For this review, take the finished solid that the model builds, in its own axes (mm). Round coordinates to 2 decimals unless told otherwise and drop trailing zeros. Write each loop counter-clockwise with the first axis right and the second up, starting at its lowest first coordinate (ties: lowest second). Pieces come first, ordered by that corner, then holes. Notation, with made-up numbers: M 23.25,15.5 L 68.25,15.5 A12 cw 68.25,31.5 Z; hole C 59.5,47 d8. An arc over 180 degrees is marked long. One line per question, with ' | ' between items.
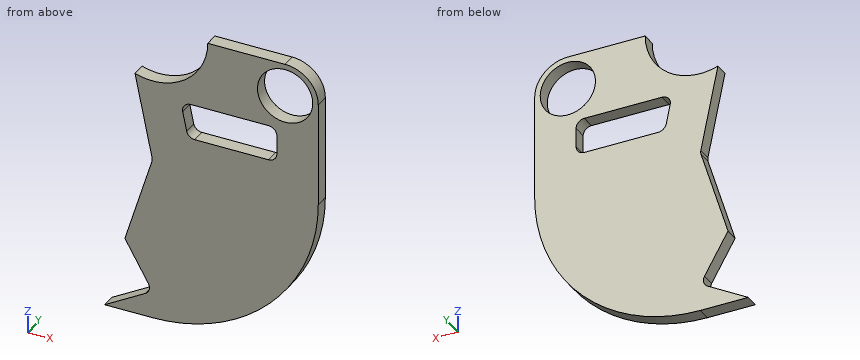
```python
from build123d import *

# Parameters (mm, degrees)
PROFILE_SKETCH_R      = 10
PROFILE_EXTRUDE_DEPTH = 5
TRAPEZOID_FILLET_R    = 3
CLAW_FILLET_R         = 3


with BuildPart() as part:
    # Profile Sketch → Profile Extrude (new body)
    with BuildSketch(Plane(origin=(0, 0, 0), x_dir=(1, 0, 0), z_dir=(0, 1, 0))):
        with BuildLine():
            Line((0, 60), (-17.320508076, 60))
            Line((-17.320508076, 60), (0, 50))
            Line((0, 50), (-10, 32.679491924))
            Line((-10, 32.679491924), (0, 0))
            Line((0, 0), (-6.333857356, -31.029437252))
            ThreePointArc((-6.333857356, -31.029437252), (11.690227818, -33.772289947), (20, -50))
            Line((20, -50), (48, -50))
            ThreePointArc((48, -50), (56.485281374, -46.485281374), (60, -38))
            Line((60, -38), (60, 0))
            ThreePointArc((60, 0), (42.426406871, 42.426406871), (0, 60))
        make_face()
        with Locations(Location((48, -38, 0), (0, 0, 270))):
            Circle(PROFILE_SKETCH_R, mode=Mode.SUBTRACT)
        Polygon((12.853812296, -12.029437252), (45, -12.029437252), (45, -25), (10.206207262, -25), align=None, mode=Mode.SUBTRACT)
    extrude(amount=PROFILE_EXTRUDE_DEPTH)

    # Trapezoid Fillet
    trapezoid_fillet_edges = [part.edges().sort_by_distance(p)[0] for p in [
        (10.206207262, 2.5, 25),
        (45, 2.5, 25),
        (45, 2.5, 12.029437252),
        (12.853812296, 2.5, 12.029437252),
    ]]
    fillet(trapezoid_fillet_edges, radius=TRAPEZOID_FILLET_R)

    # Claw Fillet
    claw_fillet_edges = [part.edges().sort_by_distance(p)[0] for p in [
        (0, 2.5, -50),
        (0, 2.5, 0),
    ]]
    fillet(claw_fillet_edges, radius=CLAW_FILLET_R)


solid = part.part
```
Item 1: Take a section at B-B (z = 19.5). Write out the cut boundary in (x, y), then the cut area to 3 significant figures.
Results:
outline: M -3.98,0 L 11.33,0 L 11.33,5 L -3.98,5 Z; M 45,0 L 60,0 L 60,5 L 45,5 Z | area: 152 mm2
Item 2: Take a section at C-C (z = -34). Write out the cut boundary in (x, y).
Results:
outline: M -9.24,0 L 49.44,0 L 49.44,5 L -9.24,5 Z
Item 3: Take a section at A-A (y = 3.45). Write out the cut boundary in (x, z).
Results:
outline: M -17.32,-60 L 0,-60 A60 ccw 60,0 L 60,38 A12 ccw 48,50 L 20,50 A20 cw -6.33,31.03 L -0.15,0.75 A3 cw -0.22,-0.73 L -10,-32.68 L -1.5,-47.4 A3 cw -2.6,-51.5 Z; hole M 10.94,21.4 L 12.36,14.43 A3 ccw 15.3,12.03 L 42,12.03 A3 ccw 45,15.03 L 45,22 A3 ccw 42,25 L 13.88,25 A3 ccw Z; hole C 48,38 d20
Item 4: To check wall thickness, follow line 1 along Z through (x, y) = (49.5, 1); line 2 along Z through (x, y) = (24, 3.5); line 3 along X through (y, z) = (3.2, 32.5). State the ranges of each line that lie inside material, in increasing order. Write a range as from..to.
Results:
line 1: -33.91..28.11, 47.89..49.91 | line 2: -54.99..12.03, 25..50 | line 3: 9.68..39.65, 56.35..60
Item 5: Insertion check: pin 1 Ø1.5 at (x, y) = (32.5, 2) entering from -Z; pin 2 Ø18 at (x, z) = (48, 38) entering from -Y; pin 3 Ø2 at (y, z) = (2, -40.5) entering from +X; pin 4 Ø2 at (x, z) = (23, -8) entering from -Y. Each pin has a flat end and moves straight along its axis. Give the tip position at first contact, or say it passes through.
Results:
pin 1: z = -50.91 | pin 2: through | pin 3: x = 45.16 | pin 4: y = 0
